For this review, use the dimensioned drawing (mm, ordinates from the lowest corner) and the shaded views. Round coordinates to 2 decimals unless told otherwise and drop trailing zeros. Write each loop counter-clockwise with the first axis right and the second up, starting at its lowest first coordinate (ties: lowest second). Pieces come first, ordered by that corner, then holes. Notation, with made-up numbers: (36.25, 65.5) - (83.25, 65.5) arc R25 ccw to (83.25, 101.5) - close; hole circle Ø8 at (25, 31.25). An arc over 180 degrees is marked (long way). Return JSON: item names as keys, results as strings.
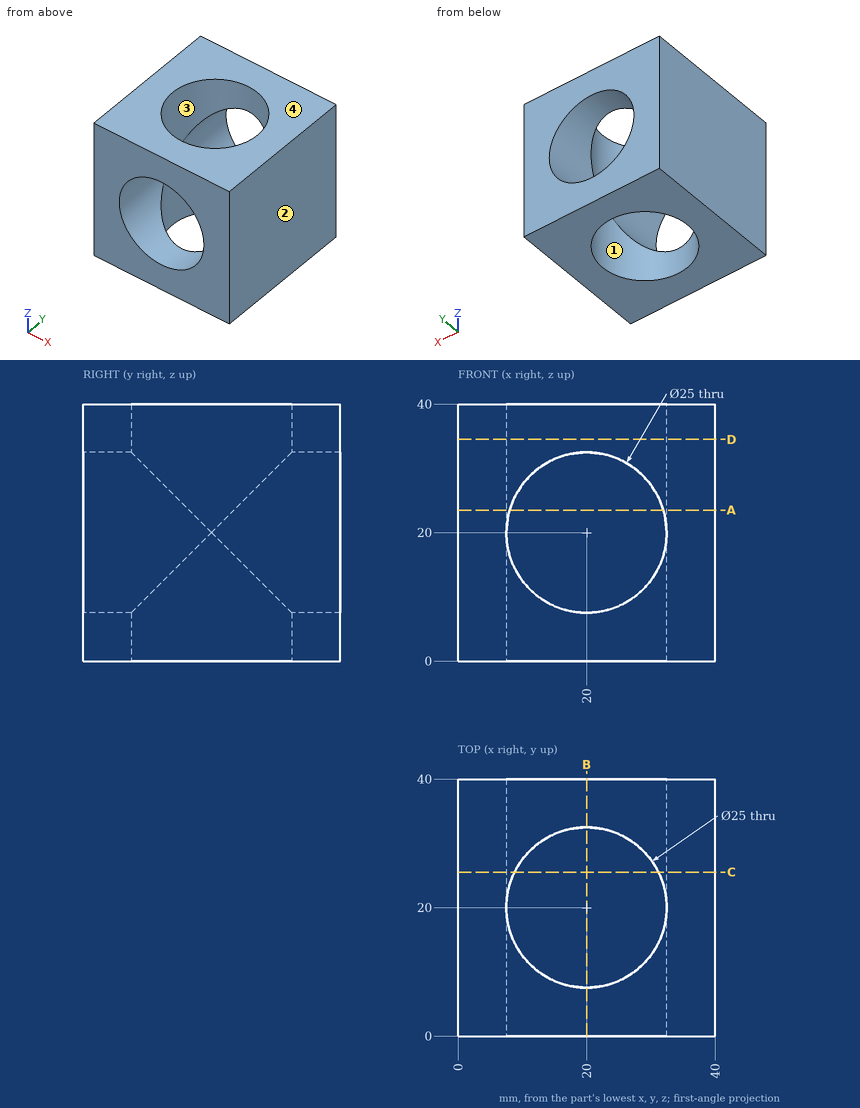
(1) Add section B-B (x = 20). Write out the cut boundary in (y, z), plus the area to 3 significant figures.
Filled in:
{"outline": "(0, 0) - (7.5, 0) - (7.5, 7.5) - (0, 7.5) - close; (0, 32.5) - (7.5, 32.5) - (7.5, 40) - (0, 40) - close; (32.5, 0) - (40, 0) - (40, 7.5) - (32.5, 7.5) - close; (32.5, 32.5) - (40, 32.5) - (40, 40) - (32.5, 40) - close", "area": "225 mm2"}
(2) Wall thickness on line 1 (Y direction, x = 20, z = 4); line 2 (X direction, y = 17, z = 16.5): over which ranges is each line inside the solid? List them lowest first.
Filled in:
{"line 1": "y = 0 to 7.5, 32.5 to 40", "line 2": "x = 0 to 7.87, 32.13 to 40"}
(3) Add section C-C (y = 25.5). Write out the cut boundary in (x, z).
Filled in:
{"outline": "(0, 0) - (8.78, 0) - (8.78, 14.5) arc R12.5 cw to (8.78, 25.5) - (8.78, 40) - (0, 40) - close; (31.22, 0) - (40, 0) - (40, 40) - (31.22, 40) - (31.22, 25.5) arc R12.5 cw to (31.22, 14.5) - close"}
(4) Clearance check with a flat-ended pin moving along its axis: pin 1 Ø20 at (x, z) = (20, 20) entering from +Y. State where the tip first meets the part, or that it passes through.
Filled in:
{"pin 1": "passes through"}
(5) Add section D-D (z = 34.5). Write out the cut boundary in (x, y).
Filled in:
{"outline": "(0, 0) - (40, 0) - (40, 40) - (0, 40) - close; hole circle Ø25 at (20, 20)"}
(6) Add section A-A (z = 23.5). Write out the cut boundary in (x, y), plus the area to 3 significant figures.
Filled in:
{"outline": "(0, 0) - (8, 0) - (8, 16.5) arc R12.5 cw to (8, 23.5) - (8, 40) - (0, 40) - close; (32, 0) - (40, 0) - (40, 40) - (32, 40) - (32, 23.5) arc R12.5 cw to (32, 16.5) - close", "area": "635 mm2"}
(7) Mouldability with a two-part tool opening along X and no side actions: class the marked faces 1, 2, 3 and 4 as released by +X, released by -X, zero draft, split by the parting line, or undercut.
Filled in:
{"face 1": "undercut", "face 2": "released by +X", "face 3": "undercut", "face 4": "zero draft"}
